Build history of the part. All positions in model axes, mm. Face numbers are marked on the shaded views. A direction names the side the tool comes from. Round coordinates to 2 decimals unless told otherwise and drop trailing zeros. Loops run counter-clockwise (first coordinate to the right, second up) from the corner with the lowest first, then second, coordinate; pieces in that order, holes last. Notation, with made-up numbers: M 73,43 L 98,43 A27 cw 98,63 Z; hole C 78.25,-38.75 d6. An arc over 180 degrees is marked long. One line per item, written item: value.
```python
from build123d import *

# Parameters (mm, degrees)
SKETCH_W        = 60
SKETCH_H        = 60
PAD_DEPTH       = 7.5
FILLET_R        = 3
SKETCH001_R     = 14.962444
POCKET_DEPTH    = 3.1
CHAMFER_SIZE    = 2
SKETCH002_R     = 14.000834
POCKET001_DEPTH = 2
FILLET001_R     = 2
SKETCH003_W     = 56.043682
SKETCH003_H     = 55.967268
SKETCH003_R     = 18
POCKET002_DEPTH = 6.5
FILLET002_R     = 1
SKETCH004_R     = 18
POCKET003_DEPTH = 4
CHAMFER001_SIZE = 2
SKETCH005_W     = 60
SKETCH005_H     = 60
SKETCH005_W_2   = 58
SKETCH005_H_2   = 57.953869
POCKET004_DEPTH = 2
FILLET003_R     = 2


with BuildPart() as part:
    # Sketch → Pad (new body)
    with BuildSketch(Plane.XY):
        Rectangle(SKETCH_W, SKETCH_H)
    extrude(amount=PAD_DEPTH)

    # Fillet
    fillet_edges = [part.edges().sort_by_distance(p)[0] for p in [
        (30, 0, 7.5),
        (0, 30, 7.5),
        (-30, 0, 7.5),
        (0, -30, 7.5),
    ]]
    fillet(fillet_edges, radius=FILLET_R)

    # Sketch001 → Pocket (cut)
    with BuildSketch(Plane.XY.offset(7.5)):
        Circle(SKETCH001_R)
    extrude(amount=-POCKET_DEPTH, mode=Mode.SUBTRACT)

    # Chamfer
    chamfer_edges = [part.edges().sort_by_distance(p)[0] for p in [
        (-14.962444, 0, 7.5),
    ]]
    chamfer(chamfer_edges, length=CHAMFER_SIZE)

    # Sketch002 → Pocket001 (cut)
    with BuildSketch(Plane.XY.offset(4.4)):
        Circle(SKETCH002_R)
    extrude(amount=-POCKET001_DEPTH, mode=Mode.SUBTRACT)

    # Fillet001
    fillet001_edges = [part.edges().sort_by_distance(p)[0] for p in [
        (-30, -30, 2.25),
        (30, -30, 2.25),
        (30, 30, 2.25),
        (-30, 30, 2.25),
    ]]
    fillet(fillet001_edges, radius=FILLET001_R)

    # Sketch003 → Pocket002 (cut)
    with BuildSketch(Plane(origin=(0, 0, 0), x_dir=(1, 0, 0), z_dir=(0, 0, -1))):
        with Locations((-0.022306, 0.060517)):
            Rectangle(SKETCH003_W, SKETCH003_H)
        Circle(SKETCH003_R, mode=Mode.SUBTRACT)
    extrude(amount=-POCKET002_DEPTH, mode=Mode.SUBTRACT)

    # Fillet002
    fillet002_edges = [part.edges().sort_by_distance(p)[0] for p in [
        (27.999535, 27.923117, 3.25),
        (-28.044147, 27.923117, 3.25),
        (-28.044147, -28.044151, 3.25),
        (27.999535, -28.044151, 3.25),
    ]]
    fillet(fillet002_edges, radius=FILLET002_R)

    # Sketch004 → Pocket003 (cut)
    with BuildSketch(Plane(origin=(0, 0, 0), x_dir=(1, 0, 0), z_dir=(0, 0, -1))):
        Circle(SKETCH004_R)
    extrude(amount=-POCKET003_DEPTH, mode=Mode.SUBTRACT)

    # Chamfer001
    chamfer001_edges = [part.edges().sort_by_distance(p)[0] for p in [
        (-18, 0, 4),
    ]]
    chamfer(chamfer001_edges, length=CHAMFER001_SIZE)

    # Sketch005 → Pocket004 (cut)
    with BuildSketch(Plane(origin=(0, 0, 0), x_dir=(1, 0, 0), z_dir=(0, 0, -1))):
        Rectangle(SKETCH005_W, SKETCH005_H)
        with Locations((0.034769, -0.002889)):
            Rectangle(SKETCH005_W_2, SKETCH005_H_2, mode=Mode.SUBTRACT)
    extrude(amount=-POCKET004_DEPTH, mode=Mode.SUBTRACT)

    # Fillet003
    fillet003_edges = [part.edges().sort_by_distance(p)[0] for p in [
        (-28.965231, 28.979824, 1),
        (-28.965231, -28.974045, 1),
        (29.034769, -28.974045, 1),
        (29.034769, 28.979824, 1),
    ]]
    fillet(fillet003_edges, radius=FILLET003_R)


solid = part.part
```
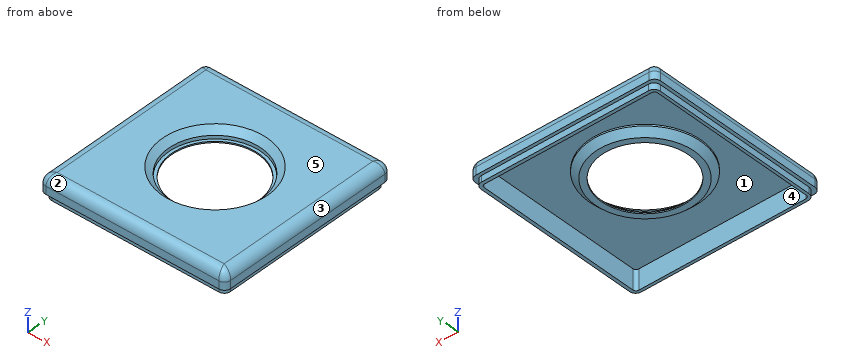
Item 1: Which spindle directions (+Z, -Z, +X, -X, +Y, -Y) get a long thin tool onto all of the face, cutting with end or side? Do the marked faces 4 and 5. Say none if no direction does.
Check values:
face 4: -Z
face 5: +Z, +X, -X, +Y, -Y
Item 2: Wall check: line 1 along Y through (x, z) = (25.5, 0.5); line 2 along Y through (x, z) = (18, 4); line 3 along X through (y, z) = (10, 2.25). Give the ranges that are in metal, low to high.
Check values:
line 1: y = -28.97 to -28.04, 27.92 to 28.98
line 2: y = -30 to -28.04, 27.92 to 30
line 3: x = -30 to -28.04, 28 to 30
Item 3: Drop flat-ended pins along their axis: P1, Ø0.6, axis at y = -2.5, z = 1, coming from the -X side; P2, Ø1.5, axis at x = -8.5, z = 6.5, coming from the -Y side; P3, Ø2, axis at y = -11, z = 0.5, coming from the +X side. Give the stop position or say it passes through.
Check values:
P1: stops at x = -28.97
P2: stops at y = -29.73
P3: stops at x = 29.03
Item 4: Pull direction X, two halves, no side cores. Call the marked faces 1, 2 and 3: pulls with the +X half, pulls with the -X half, needs draft (parallel to the pull), parting line crosses it, or undercut.
Check values:
face 1: undercut
face 2: needs draft
face 3: pulls with the +X half
Item 5: Slice it at A-A, the plane z = 1. Give the cut face in (x, y).
Check values:
outline: M -28.97,-26.97 A2 ccw -26.97,-28.97 L 27.03,-28.97 A2 ccw 29.03,-26.97 L 29.03,26.98 A2 ccw 27.03,28.98 L -26.97,28.98 A2 ccw -28.97,26.98 Z; hole M -28.04,-27.04 A1 ccw -27.04,-28.04 L 27,-28.04 A1 ccw 28,-27.04 L 28,26.92 A1 ccw 27,27.92 L -27.04,27.92 A1 ccw -28.04,26.92 Z
